For this review, take the finished solid that the model builds, in its own axes (mm). A direction names the side the tool comes from. Give positions to 0.01 mm unless a question says otherwise; leave off trailing zeros. Loops run counter-clockwise (first coordinate to the right, second up) from the corner with the lowest first, then second, coordinate; pieces in that order, holes last. Notation, with made-up numbers: (6, 38.5) - (26, 38.5) arc R18 ccw to (26, 60.5) - close; hole circle Ø9 at (-31.5, 25). An arc over 180 degrees is marked (long way). Answer in a Markdown table with one row per item.
```python
from build123d import *

# Parameters (mm, degrees)
F0_R     = 12
F1_DEPTH = 63
F2_R     = 15
F2_R_2   = 12
F3_DEPTH = 8
F4_R     = 10
F5_DEPTH = 25
F6_R     = 3
F8_DEPTH = 31.2849479744


with BuildPart() as f1:
    # F0 (on Front) → F1 (new body)
    with BuildSketch(Plane.XZ):
        with Locations((18.5694117099, 16.2839479744)):
            Circle(F0_R)
    extrude(amount=F1_DEPTH)

    # F2 (on face) → F3 (join)
    with BuildSketch(Plane(origin=(0, 0, 0), x_dir=(-1, 0, 0), z_dir=(0, 1, 0))):
        with Locations((-18.5694117099, 16.2839479744)):
            Circle(F2_R)
        with Locations((-18.5694117099, 16.2839479744)):
            Circle(F2_R_2, mode=Mode.SUBTRACT)
        with Locations((-18.5694117099, 16.2839479744)):
            Circle(F2_R_2)
    extrude(amount=F3_DEPTH)

    # F4 (on face) → F5 (join)
    with BuildSketch(Plane(origin=(0, 8, 0), x_dir=(-1, 0, 0), z_dir=(0, 1, 0))):
        with Locations((-18.5694117099, 16.2839479744)):
            Circle(F4_R)
    extrude(amount=F5_DEPTH)

    # F6
    f6_edges = [f1.edges().sort_by_distance(p)[0] for p in [
        (33.569412, 8, 16.283948),
    ]]
    fillet(f6_edges, radius=F6_R)

    # F7 (on Top) → F8 (cut, through all)
    with BuildSketch(Plane.XY):
        Polygon((21.912544474, -4.9977113605), (18.912544474, -4.9977113605), (15.912544474, -4.9977113605), (15.912544474, -30.9977113605), (18.912544474, -30.9977113605), (21.912544474, -30.9977113605), align=None)
    extrude(amount=F8_DEPTH, mode=Mode.SUBTRACT)


solid = f1.part
```
1. For faces 4 (the face through (30.015, -31.059, 19.888)), 5 (the face through (15.913, -18, 16)), 6 (the face through (19, 33, 16)), 7 (the face through (19.87, 20.32, 26.2)), list the 3-axis set-ups (+Z, -Z, +X, -X, +Y, -Y) from which the entire face can be reached by the end or side of a thin tool; tool diameter is ignored.
Values:
| item | result |
|---|---|
| face 4 | -Y |
| face 5 | +Z, -Z |
| face 6 | +Z, -Z, +X, -X, +Y |
| face 7 | +Y |
2. Mouldability with a two-part tool opening along X and no side actions: class faces 1 (the face through (19, -4.998, 16)), 2 (the face through (18, -63, 16)), 3 (the face through (21.82, 2.46, 1.64)) as released by +X, released by -X, zero draft, split by the parting line, or undercut.
Values:
| item | result |
|---|---|
| face 1 | undercut |
| face 2 | zero draft |
| face 3 | split by the parting line |
3. We need section B-B, the plane y = -49. Give the boundary of the cut face in (x, z), and give its area (3 significant figures).
Values:
| item | result |
|---|---|
| outline | circle Ø24 at (18.57, 16.28) |
| area | 452 mm^2 |
4. We need section A-A, the plane y = -22. Give the boundary of the cut face in (x, z).
Values:
| item | result |
|---|---|
| outline | (15.91, 4.58) - (15.91, 27.99) arc R12 ccw to start; (21.91, 4.76) arc R12 ccw to (21.91, 27.81) - close |
5. Wall thickness on line 1 (Y direction, x = 20.5, z = 12); line 2 (Y direction, x = 26, z = 6.75); line 3 (Y direction, x = 26, z = 8): over which ranges is each line inside the solid? List them lowest first. Write a range as [from, to].
Values:
| item | result |
|---|---|
| line 1 | y = [-63, -31], [-5, 33] |
| line 2 | y = [0, 8] |
| line 3 | y = [-63, 8] |
6. Clearance check with flat-ended pins moving along their axes: pin 1 (6 mm diameter, centred on x = 13.5, y = -31, fed in from +Z); pin 2 (4 mm diameter, centred on x = 22, y = -25.5, fed in from +Z); pin 3 (7 mm diameter, centred on y = -13.5, z = 18, fed in from +X). State where each tip first meets the part, or that it passes through.
Values:
| item | result |
|---|---|
| pin 1 | stops at z = 28.1 |
| pin 2 | stops at z = 27.81 |
| pin 3 | stops at x = 30.57 |
7. We need section C-C, the plane y = 2. Give the boundary of the cut face in (x, z), and give its area (3 significant figures).
Values:
| item | result |
|---|---|
| outline | circle Ø30 at (18.57, 16.28) |
| area | 707 mm^2 |
